Read the model definition and answer for the solid it produces. Units are mm, in the model's axes. Give positions to 0.01 mm unless a question says otherwise; leave off trailing zeros. Order: outer loops, then holes, each group sorted by start corner. A loop starts at its lowest first (then second) coordinate and runs counter-clockwise, first axis right, second up.
Item 1: A cutting plane is placed at A-A (y = 1.6). Write down the section's boundary in (x, z).
Item 2: Find the intervals of material crossed by line 1 along Z through (x, y) = (0, 1.75); line 2 along X through (y, z) = (1.7, 0); line 3 along X through (y, z) = (1.25, 10.16), in increasing order.
Item 3: A cutting plane is placed at B-B (z = 17). Write down the section's boundary in (x, y) (3 decimals), plus the area to 3 significant figures.
Item 4: Given pin 1 Ø1 at (y, z) = (1, 2.5) entering from -X; pin 2 Ø1.6 at (y, z) = (1.5, 1.5) entering from +X; pin 3 Ø5 at (x, z) = (0, 0) entering from +Y; pin 4 Ø1.6 at (x, y) = (36.5, 1) entering from +Z, each flat-ended and moving along its own axis, determine where each tip first touches the part or whether it passes through.
from build123d import *

# Parameters (mm, degrees)
SKETCH1_W                            = 70.104
SKETCH1_H                            = 38.1
BOSS_EXTRUDE1_DEPTH                  = 3.175
SKETCH2_W                            = 3.2258
SKETCH2_H                            = 6.35
BOSS_EXTRUDE2_DEPTH                  = 3.175
SKETCH4_R                            = 2.667
SKETCH4_R_2                          = 0.4445
CUT_FOR_SERVO_HORN_MOUNT_HOLES_DEPTH = 4.175


with BuildPart() as part:
    # Sketch1 → Boss-Extrude1 (new body)
    with BuildSketch(Plane(origin=(0, 0, 0), x_dir=(1, 0, 0), z_dir=(0, 1, 0))):
        Rectangle(SKETCH1_W, SKETCH1_H)
    extrude(amount=BOSS_EXTRUDE1_DEPTH)

    # Sketch2 → Boss-Extrude2 (add)
    with BuildSketch(Plane(origin=(0, 3.175, 0), x_dir=(1, 0, 0), z_dir=(0, 1, 0))):
        with Locations((36.6649, 9.525)):
            Rectangle(SKETCH2_W, SKETCH2_H)
        with Locations((36.6649, -9.525)):
            Rectangle(SKETCH2_W, SKETCH2_H)
    boss_extrude2 = extrude(amount=-BOSS_EXTRUDE2_DEPTH)

    # Mirror1: Boss-Extrude2 across plane
    add(boss_extrude2.mirror(Plane(origin=(0, 0, 0), x_dir=(0, 0, 1), z_dir=(1, 0, 0))))

    # Sketch4 → cut for servo horn mount holes (cut, through all)
    with BuildSketch(Plane(origin=(0, 3.175, 0), x_dir=(1, 0, 0), z_dir=(0, 1, 0))):
        Circle(SKETCH4_R)
        with Locations((0, 10.16)):
            Circle(SKETCH4_R_2)
        with Locations((10.16, 0)):
            Circle(SKETCH4_R_2)
        with Locations((0, -10.16)):
            Circle(SKETCH4_R_2)
        with Locations((-10.16, 0)):
            Circle(SKETCH4_R_2)
    extrude(amount=-CUT_FOR_SERVO_HORN_MOUNT_HOLES_DEPTH, mode=Mode.SUBTRACT)


solid = part.part
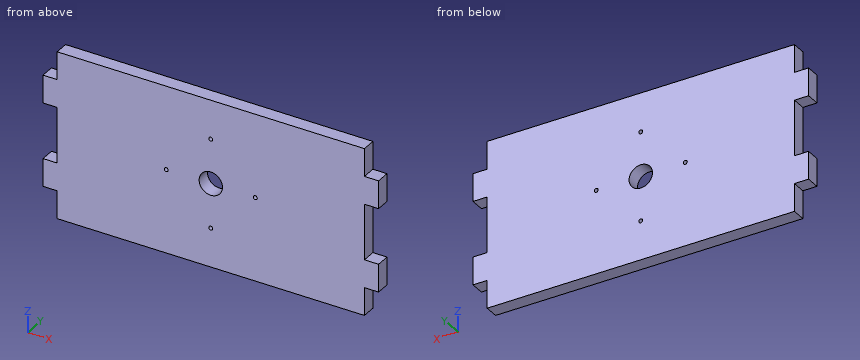
Response values:
1. outline: (-38.28, -12.7) - (-35.05, -12.7) - (-35.05, -19.05) - (35.05, -19.05) - (35.05, -12.7) - (38.28, -12.7) - (38.28, -6.35) - (35.05, -6.35) - (35.05, 6.35) - (38.28, 6.35) - (38.28, 12.7) - (35.05, 12.7) - (35.05, 19.05) - (-35.05, 19.05) - (-35.05, 12.7) - (-38.28, 12.7) - (-38.28, 6.35) - (-35.05, 6.35) - (-35.05, -6.35) - (-38.28, -6.35) - close; hole circle Ø0.89 at (-10.16, 0); hole circle Ø5.33 at (0, 0); hole circle Ø0.89 at (0, -10.16); hole circle Ø0.89 at (0, 10.16); hole circle Ø0.89 at (10.16, 0)
2. line 1: z = -19.05 to -10.6, -9.72 to -2.67, 2.67 to 9.72, 10.6 to 19.05
2. line 2: x = -35.05 to -10.6, -9.72 to -2.67, 2.67 to 9.72, 10.6 to 35.05
2. line 3: x = -38.28 to -0.44, 0.44 to 38.28
3. outline: (-35.052, 0) - (35.052, 0) - (35.052, 3.175) - (-35.052, 3.175) - close
3. area: 223 mm2
4. pin 1: stops at x = -35.05
4. pin 2: stops at x = 35.05
4. pin 3: passes through
4. pin 4: stops at z = 12.7
